Source: CAD feature listing. Evaluate the final solid. Frame: model axes, mm. Face numbers are marked on the shaded views. A direction names the side the tool comes from. Give positions to 0.01 mm unless a question says otherwise; leave off trailing zeros. Write each loop counter-clockwise with the first axis right and the second up, starting at its lowest first coordinate (ties: lowest second). Pieces come first, ordered by that corner, then holes. Notation, with made-up numbers: (72, 84) -> (98, 84) arc R16 ccw to (98, 99) -> close; hole circle Ø3 at (8, 54.25). An arc over 180 degrees is marked (long way). Use a Markdown table: item, result. Add a question column.
```python
from build123d import *

# Parameters (mm, degrees)
F0_R            = 42.5
F0_R_2          = 11
F1_DEPTH        = 6
F3_DEPTH        = 25
F3_COPIES_COUNT = 3
F4_R            = 5


# Not quite as in the source:
# - a pattern or mirror of a feature is missing from the dataset's text; its kind, count and spacing are read off the source's solid


with BuildPart() as f1:
    # F0 (on Top) → F1 (new body)
    with BuildSketch(Plane.XY):
        Circle(F0_R)
        with Locations((0, -25.9807621135)):
            Circle(F0_R_2, mode=Mode.SUBTRACT)
        with Locations((-22.5, 12.9903810568)):
            Circle(F0_R_2, mode=Mode.SUBTRACT)
        Circle(F0_R_2, mode=Mode.SUBTRACT)
        with Locations((22.5, 12.9903810568)):
            Circle(F0_R_2, mode=Mode.SUBTRACT)
    extrude(amount=F1_DEPTH)

    # F2 (on face) → F3 (cut)
    with BuildSketch(Plane.XY.offset(6)):
        with BuildLine():
            Line((11.9734825652, -6.9128933822), (26.9537505179, -32.8594785872))
            ThreePointArc((26.9537505179, -32.8594785872), (36.8060796608, -21.25), (41.9340184705, -6.9128933822))
            Line((41.9340184705, -6.9128933822), (11.9734825652, -6.9128933822))
        make_face()
    f3 = extrude(amount=-F3_DEPTH, mode=Mode.SUBTRACT)

    # F3_copies: F3 ×3 about axis
    f3_copies_axis = Axis((0, 0, 0), (0, 0, 1))
    for i in range(1, F3_COPIES_COUNT):
        add(f3.rotate(f3_copies_axis, i * 360 / F3_COPIES_COUNT), mode=Mode.SUBTRACT)

    # F4
    f4_edges = [f1.edges().sort_by_distance(p)[0] for p in [
        (11.973483, -6.912893, 3),
        (0, 13.825787, 3),
        (-11.973483, -6.912893, 3),
    ]]
    fillet(f4_edges, radius=F4_R)


solid = f1.part
```
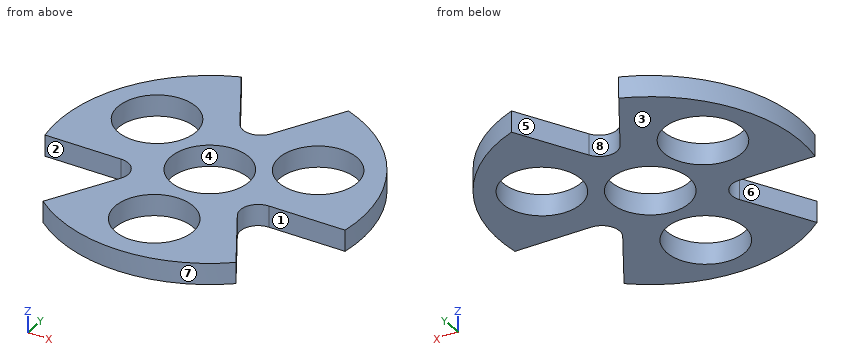
(1) Cut plane C-C on x = -13.5. Return the cut outline in (y, z).
(2) Material intervals for L1, parallel to Y at x = 22.5, z = 3.2; L2, parallel to Y at x = -5.5, z = 5.5; L3, parallel to X at y = 12, z = 5, sorted ascending.
(3) Access query for the marked faces 1, 2, 3, 4 and 5. Directions: +Z, -Z, +X, -X, +Y, -Y. A direction counts if a zero-diameter tool reaches every point of the face in a straight line with its end or side. Return the directions, or none.
(4) First-contact query: pin 1 Ø3 at (x, z) = (-35.5, 2.5) entering from -Y; pin 2 Ø3 at (x, z) = (9.5, 5.5) entering from +Y; pin 3 Ø3 at (y, z) = (-21.5, 5) entering from -X. Flat tips, straight axial feed; report the tip coordinate or a pass-through.
(5) Cut plane D-D on z = 4. Return the cut outline in (x, y), then the cut area to 3 significant figures.
(6) Mould query, pull axis Y, two halves, no side actions, for the marked faces 6, 7 and 8. Classes: +Y half, -Y half, draft (parallel to the pull), parting line (faces both ways), or undercut.
(7) Cut plane A-A on x = 0. Return the cut outline in (y, z), then the cut area to 3 significant figures.
(8) Cut plane B-B on y = 0. Return the cut outline in (x, z), then the cut area to 3 significant figures.
Output:
| question | item | result |
|---|---|---|
| 1 | outline | (-40.3, 0) -> (6.67, 0) -> (6.67, 6) -> (-40.3, 6) -> close; (19.31, 0) -> (37.21, 0) -> (37.21, 6) -> (19.31, 6) -> close |
| 2 | L1 | -36.06 to -25.15, -6.91 to 1.99, 23.99 to 36.06 |
| 2 | L2 | -42.14 to -35.51, -16.45 to -9.53, 9.53 to 23.35 |
| 2 | L3 | -40.77 to -33.46, -11.54 to 11.54, 33.46 to 40.77 |
| 3 | face 1 | +Z, -Z, +X |
| 3 | face 2 | +Z, -Z, -X |
| 3 | face 3 | -Z, +X, -X, +Y, -Y |
| 3 | face 4 | +Z, -Z |
| 3 | face 5 | +Z, -Z, +Y |
| 4 | pin 1 | y = -6.91 |
| 4 | pin 2 | y = 32.88 |
| 4 | pin 3 | x = -21.26 |
| 5 | outline | (-41.93, -6.91) -> (-20.63, -6.91) arc R5 cw to (-16.3, -14.41) -> (-26.95, -32.86) arc R42.5 ccw to (26.95, -32.86) -> (16.3, -14.41) arc R5 cw to (20.63, -6.91) -> (41.93, -6.91) arc R42.5 ccw to (14.98, 39.77) -> (4.33, 21.33) arc R5 cw to (-4.33, 21.33) -> (-14.98, 39.77) arc R42.5 ccw to start; hole circle Ø22 at (-22.5, 12.99); hole circle Ø22 at (0, -25.98); hole circle Ø22 at (0, 0); hole circle Ø22 at (22.5, 12.99) |
| 5 | area | 2,870 mm^2 |
| 6 | face 6 | undercut |
| 6 | face 7 | -Y half |
| 6 | face 8 | +Y half |
| 7 | outline | (-42.5, 0) -> (-36.98, 0) -> (-36.98, 6) -> (-42.5, 6) -> close; (-14.98, 0) -> (-11, 0) -> (-11, 6) -> (-14.98, 6) -> close; (11, 0) -> (18.83, 0) -> (18.83, 6) -> (11, 6) -> close |
| 7 | area | 104 mm^2 |
| 8 | outline | (-42.5, 0) -> (-11, 0) -> (-11, 6) -> (-42.5, 6) -> close; (11, 0) -> (42.5, 0) -> (42.5, 6) -> (11, 6) -> close |
| 8 | area | 378 mm^2 |
